```python
from build123d import *

# Parameters (mm, degrees)
SKETCH_R      = 32.5
SKETCH_R_2    = 25
PAD_DEPTH     = 7
SKETCH001_R   = 31
SKETCH001_R_2 = 26.5
POCKET_DEPTH  = 1
CHAMFER_SIZE  = 0.5


with BuildPart() as part:
    # Sketch → Pad (new body)
    with BuildSketch(Plane.XY.offset(-3.5)):
        Circle(SKETCH_R)
        Circle(SKETCH_R_2, mode=Mode.SUBTRACT)
    extrude(amount=PAD_DEPTH)

    # Sketch001 (on Face4 of Pad) → Pocket (cut)
    with BuildSketch(Plane.XY.offset(3.5)):
        Circle(SKETCH001_R)
        Circle(SKETCH001_R_2, mode=Mode.SUBTRACT)
    pocket = extrude(amount=-POCKET_DEPTH, mode=Mode.SUBTRACT)

    # Mirrored: Pocket across XY
    add(pocket.mirror(Plane.XY), mode=Mode.SUBTRACT)

    # Chamfer
    chamfer_edges = [part.edges().sort_by_distance(p)[0] for p in [
        (-32.5, 0, 3.5),
        (-32.5, 0, -3.5),
        (-25, 0, 3.5),
        (-25, 0, -3.5),
    ]]
    chamfer(chamfer_edges, length=CHAMFER_SIZE)


solid = part.part
```
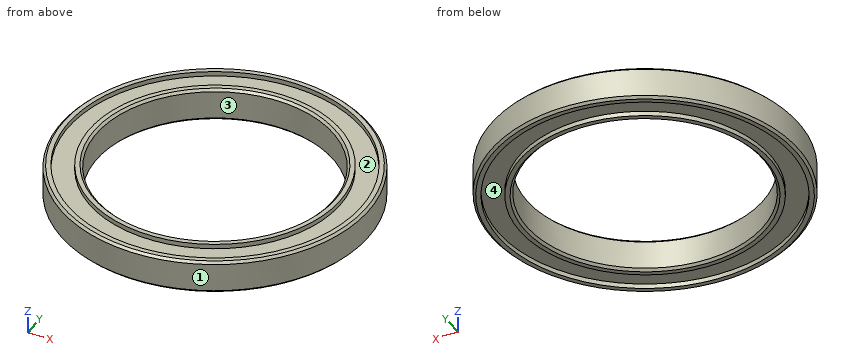
Design review of the part built by this model. Coordinates are the model's own, in mm. Face numbers are marked on the shaded views. A direction names the side the tool comes from. Give positions to 0.01 mm unless a question says otherwise; leave off trailing zeros. Loops run counter-clockwise (first coordinate to the right, second up) from the corner with the lowest first, then second, coordinate; pieces in that order, holes last. Notation, with made-up numbers: (27, -34) -> (31, -34) arc R16 ccw to (31, -26) -> close; hole circle Ø11 at (12, 32.5). An arc over 180 degrees is marked (long way). One line per item, written item: value.
Q1. Draft analysis for pull direction X (two halves, no side actions). For the marked faces 1 and 2, state which applies: pulls with the +X half, pulls with the -X half, needs draft (parallel to the pull), parting line crosses it, or undercut.
Numbers:
face 1: parting line crosses it
face 2: undercut
Q2. For L1, parallel to Y at x = 0, z = -2.75; L2, parallel to Y at x = 0, z = -1.35; L3, parallel to X at y = 8.5, z = 3, list the stretches that pass through material, from the lowest coordinate up.
Numbers:
L1: y = -32.5 to -31, -26.5 to -25, 25 to 26.5, 31 to 32.5
L2: y = -32.5 to -25, 25 to 32.5
L3: x = -31.37 to -29.81, -25.1 to -23.51, 23.51 to 25.1, 29.81 to 31.37
Q3. We need section C-C on z = -0.75. Give the boundary of the cut face in (x, y).
Numbers:
outline: circle Ø65 at (0, 0); hole circle Ø50 at (0, 0)
Q4. Machinability: for the marked faces 3 and 4, which of the approach directions +Z, -Z, +X, -X, +Y, -Y give a long, thin tool a straight path to every point of the face, cutting with its end or side? Answer none if there is none.
Numbers:
face 3: +Z, -Z
face 4: -Z
Q5. For pin 1 Ø4 at (x, z) = (-25, -2) entering from -Y; pin 2 Ø2 at (x, z) = (-20, -1) entering from +Y; pin 3 Ø3 at (x, z) = (-4, -1.5) entering from -Y; pin 4 Ø8 at (x, y) = (15, -19.5) entering from +Z, all flat-tipped, find the tip position at first contact; note any pin that passes through.
Numbers:
pin 1: stops at y = -22.96
pin 2: stops at y = 26.37
pin 3: stops at y = -32.4
pin 4: stops at z = 3.5
